from build123d import *

# Parameters (mm, degrees)
F1_R           = 12.826844
F2_DEPTH       = 76.2
F2_DEPTH_BACK  = 76.2
F3_D           = 12.7
F4_D           = 12.7
F5_W           = 25.60015
F5_H           = 53.179082
F6_DEPTH       = 6.35
F8_R           = 12.706951
F9_DEPTH       = 2.54
F11_D          = 6.35
F10_R          = 6.772229
F12_DEPTH      = 50.8
F12_DEPTH_BACK = 50.8


with BuildPart() as f2:
    # F1 (on Front) → F2 (new body, two sides)
    with BuildSketch(Plane.XZ) as f2_sk:
        Circle(F1_R)
    extrude(amount=F2_DEPTH)
    extrude(f2_sk.sketch, amount=-F2_DEPTH_BACK)

    # F3 (through all)
    with Locations(Plane.XZ):
        with Locations((0, 0)):
            Hole(F3_D / 2)

    # F4 (through all)
    with Locations(Plane(origin=(0, 0, 0), x_dir=(1, 0, 0), z_dir=(0, 1, 0))):
        with Locations((0, 0)):
            Hole(F4_D / 2)

    # F5 (on offset) → F6 (join)
    with BuildSketch(Plane.XZ.offset(76.2)):
        Rectangle(F5_W, F5_H)
    extrude(amount=F6_DEPTH)

    # F8 (on offset) → F9 (join)
    with BuildSketch(Plane.XZ.offset(-76.2)):
        Circle(F8_R)
    extrude(amount=-F9_DEPTH)

    # F11 (through all)
    with Locations(Plane.YZ):
        with Locations((0, 0)):
            Hole(F11_D / 2)

    # F10 (on Right) → F12 (cut, two sides)
    with BuildSketch(Plane.YZ) as f12_sk:
        Circle(F10_R)
    extrude(amount=F12_DEPTH, mode=Mode.SUBTRACT)
    extrude(f12_sk.sketch, amount=-F12_DEPTH_BACK, mode=Mode.SUBTRACT)


solid = f2.part
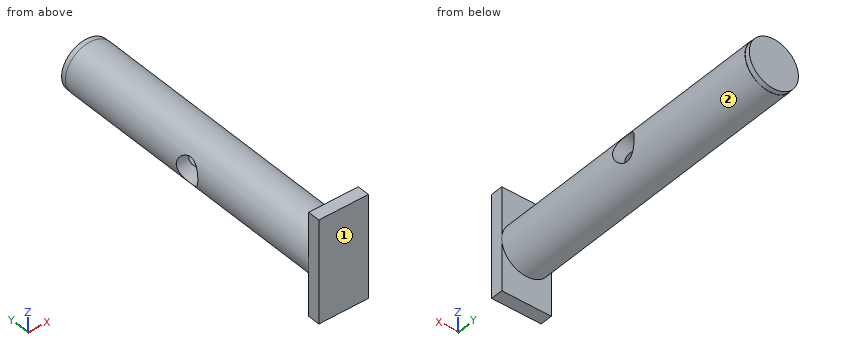
Design review of the part built by this model. Coordinates are the model's own, in mm. Face numbers are marked on the shaded views. A direction names the side the tool comes from. Coordinates: 2 decimals unless noted, no trailing zeros. Loops run counter-clockwise (first coordinate to the right, second up) from the corner with the lowest first, then second, coordinate; pieces in that order, holes last. Notation, with made-up numbers: M 59,40.5 L 106,40.5 A31 ccw 106,66.5 Z; hole C -3.75,36.5 d8. An arc over 180 degrees is marked long. Use one line per item in the form item = value.
(1) For line 1 along X through (y, z) = (40, 0); line 2 along Y through (x, z) = (6.25, 24); line 3 along Y through (x, z) = (2.5, 12.5), list the stretches that pass through material, from the lowest coordinate up. Write a range as from..to.
Return value:
line_1 = -12.83..-6.35, 6.35..12.83
line_2 = -82.55..-76.2
line_3 = -82.55..76.2
(2) Clearance check with flat-ended pins moving along their axes: P1, Ø5, axis at y = -80, z = 7.5, coming from the +X side; P2, Ø1, axis at x = -1, y = -10, coming from the -Z side; P3, Ø10, axis at x = -7, y = 42, coming from the +Z side. State where each tip first meets the part, or that it passes through.
Return value:
P1 = 12.8
P2 = -12.82
P3 = 12.67
(3) For the marked faces 1 and 2, list the 3-axis set-ups (+Z, -Z, +X, -X, +Y, -Y) from which the entire face can be reached by the end or side of a thin tool; tool diameter is ignored.
Return value:
face_1 = +Z, -Z, +X, -X, -Y
face_2 = +Y
(4) Consider section A-A (x = 4.25). Write out the cut boundary in (y, z), and give its area (3 significant figures).
Return value:
outline = M -82.55,-26.59 L -76.2,-26.59 L -76.2,-12.1 L 76.2,-12.1 L 76.2,-11.98 L 78.74,-11.98 L 78.74,11.98 L 76.2,11.98 L 76.2,12.1 L -76.2,12.1 L -76.2,26.59 L -82.55,26.59 Z; hole M -76.2,-4.72 L -4.86,-4.72 A6.77 ccw 4.86,-4.72 L 76.2,-4.72 L 76.2,4.72 L 4.86,4.72 A6.77 ccw -4.86,4.72 L -76.2,4.72 Z
area = 2,620 mm2
(5) Consider section B-B (y = -4). Write out the cut boundary in (x, z), and give its area (3 significant figures).
Return value:
outline = M -11.6,-5.46 A12.83 ccw 11.6,-5.46 L 3.23,-5.46 A6.35 cw -3.23,-5.46 Z; M -11.6,5.46 L -3.23,5.46 A6.35 cw 3.23,5.46 L 11.6,5.46 A12.83 ccw Z
area = 237 mm2
(6) Consider section C-C (y = -38). Write out the cut boundary in (x, z), and give its area (3 significant figures).
Return value:
outline = C 0,0 d25.65; hole C 0,0 d12.7
area = 390 mm2
(7) Consider section D-D (x = -4.75). Write out the cut boundary in (y, z).
Return value:
outline = M -82.55,-26.59 L -76.2,-26.59 L -76.2,-11.91 L 76.2,-11.91 L 76.2,-11.79 L 78.74,-11.79 L 78.74,11.79 L 76.2,11.79 L 76.2,11.91 L -76.2,11.91 L -76.2,26.59 L -82.55,26.59 Z; hole M -76.2,-4.21 L -5.3,-4.21 A6.77 ccw 5.3,-4.21 L 76.2,-4.21 L 76.2,4.21 L 5.3,4.21 A6.77 ccw -5.3,4.21 L -76.2,4.21 Z
